Model file for the job. Use its own axes, mm. A direction names the side the tool comes from. Round coordinates to 2 decimals unless told otherwise and drop trailing zeros. Write each loop counter-clockwise with the first axis right and the second up, starting at its lowest first coordinate (ties: lowest second). Pieces come first, ordered by that corner, then holes. Notation, with made-up numbers: (30, 53.5) - (70, 53.5) arc R8 ccw to (70, 62.5) - close; hole circle Ø7 at (-24, 49). An arc over 180 degrees is marked (long way). One line per item, written item: value.
Autodesk Inventor part; units mm, degrees
ref_plane "作業平面1" through (2.15, -10, 1000) normal (0, 0, 1) x (1, 0, 0)
ref_plane "YZ Plane" through (0, 0, 0) normal (1, 0, 0) x (0, 1, 0)
ref_plane "XZ Plane" through (0, 0, 0) normal (0, 1, 0) x (-1, 0, 0)
ref_plane "作業平面1" through (2.15, -10, 1000) normal (0, 0, 1) x (1, 0, 0)
sketch "スケッチ1" plane through (2.15, -10, 1000) normal (0, 0, 1) x (1, 0, 0)
  line L0 (6.35, 12.15) -> (7.85, 12.15)
  line L1 (7.85, 12.15) -> (7.85, 19.4936)
  arc A0 (7.85, 19.4936) -> (7.3372, 19.9934) centre (7.35, 19.4936) ccw
  arc A1 (7.3372, 19.9934) -> (-12.1434, 0.5128) centre (7.85, 0) ccw
  arc A2 (-12.1434, 0.5128) -> (-11.6436, 0) centre (-11.6436, 0.5) ccw
  line L2 (-11.6436, 0) -> (-4.3, 0)
  line L3 (-4.3, 0) -> (-4.3, 1.5)
  line L4 (-4.3, 1.5) -> (-6.3, 1.5)
  line L5 (-6.3, 1.5) -> (-6.3, 5.2)
  line L6 (-6.3, 5.2) -> (-4.3, 5.2)
  line L7 (-4.3, 5.2) -> (-4.3, 7)
  line L8 (-4.3, 7) -> (0, 7)
  line L9 (0, 7) -> (0, 5.2)
  line L10 (0, 5.2) -> (2, 5.2)
  line L11 (2, 5.2) -> (2, 1.5)
  line L12 (2, 1.5) -> (0, 1.5)
  line L13 (0, 1.5) -> (0, 0)
  line L14 (0, 0) -> (7.35, 0)
  arc A3 (7.35, 0) -> (7.85, 0.5) centre (7.35, 0.5) ccw
  line L15 (7.85, 0.5) -> (7.85, 7.85)
  line L16 (7.85, 7.85) -> (6.35, 7.85)
  line L17 (6.35, 7.85) -> (6.35, 5.85)
  line L18 (6.35, 5.85) -> (2.65, 5.85)
  line L19 (2.65, 5.85) -> (2.65, 7.85)
  line L20 (2.65, 7.85) -> (0.85, 7.85)
  line L21 (0.85, 7.85) -> (0.85, 12.15)
  line L22 (0.85, 12.15) -> (2.65, 12.15)
  line L23 (2.65, 12.15) -> (2.65, 14.15)
  line L24 (2.65, 14.15) -> (6.35, 14.15)
  line L25 (6.35, 14.15) -> (6.35, 12.15)
  circle A4 centre (4.85, 3) radius 2
  circle A5 centre (-9.15, 3) radius 2
  circle A6 centre (4.85, 17) radius 2
  circle A7 centre (-2.15, 10) radius 1.65
extrude "押し出し1" add sketch "スケッチ1" along normal blind 40
properties part number "AFSR-2020-4-1000"
1. Tool access for faces 1 (the face through (4.8, 3, 1020)), 2 (the face through (2.15, -4, 1020)), 3 (the face through (4, -2.15, 1020)), 4 (the face through (2, 0, 1000)): list every direction of +Z, -Z, +X, -X, +Y, -Y with a clear straight run to the whole face (end or side of a thin tool).
Report:
face 1: +Z, -Z
face 2: +Z, -Z, -Y
face 3: +Z, -Z, +X
face 4: -Z, +X, -X, +Y, -Y
2. Band-saw the part on C-C on y = 0. Write the cut outline in (x, z), plus the area to 3 significant figures.
Report:
outline: (-7.32, 1000) - (-1.65, 1000) - (-1.65, 1040) - (-7.32, 1040) - close; (1.65, 1000) - (3, 1000) - (3, 1040) - (1.65, 1040) - close
area: 281 mm²
3. Band-saw the part on B-B on x = 7. Write the cut outline in (y, z).
Report:
outline: (-10, 1000) - (-9, 1000) - (-9, 1040) - (-10, 1040) - close; (-5, 1000) - (-4.15, 1000) - (-4.15, 1040) - (-5, 1040) - close; (4.15, 1000) - (5, 1000) - (5, 1040) - (4.15, 1040) - close; (9, 1000) - (9.77, 1000) - (9.77, 1040) - (9, 1040) - close
4. Band-saw the part on D-D on y = -7. Write the cut outline in (x, z).
Report:
outline: (-9.77, 1000) - (-9, 1000) - (-9, 1040) - (-9.77, 1040) - close; (-5, 1000) - (-4.15, 1000) - (-4.15, 1040) - (-5, 1040) - close; (4.15, 1000) - (5, 1000) - (5, 1040) - (4.15, 1040) - close; (9, 1000) - (10, 1000) - (10, 1040) - (9, 1040) - close
5. Band-saw the part on A-A on z = 1017.5. State how many separate pieces and enclosed holes the cut face has, plus the area to 3 significant figures.
Report:
separate pieces: 1
enclosed holes: 4
area: 178 mm²
6. Drop flat-ended pins along their axis: pin 1 (5 mm diameter, centred on y = -4, z = 1025.5, fed in from -X); pin 2 (1.4 mm diameter, centred on x = 4, z = 1030, fed in from +Y); pin 3 (1.6 mm diameter, centred on x = 2.5, z = 1027, fed in from +Y). Give the stop position or say it passes through.
Report:
pin 1: x = -9.69
pin 2: y = 9.28
pin 3: y = 8.84
7. Mould opens along X. For faces 5 (the face through (2.15, -9, 1020)), 6 (the face through (9, -2.15, 1020)), 7 (the face through (4.8, -3, 1020)), 8 (the face through (3, 0, 1020)) say: released by +X, released by -X, zero draft, split by the parting line, or undercut.
Report:
face 5: undercut
face 6: zero draft
face 7: undercut
face 8: released by +X
8. Wall check: probe 1 along Y at (x, z) = (7, 1009.5); probe 2 along Y at (x, z) = (7.5, 1036.5); probe 3 along X at (y, z) = (-7.75, 1020). Give the ranges that are in metal, low to high. Write a range as [from, to].
Report:
probe 1: [-10, -9], [-5, -4.15], [4.15, 5], [9, 9.77]
probe 2: [-10, -8.94], [-5.06, -4.15], [4.15, 5.06], [8.94, 9.84]
probe 3: [-9.87, -8.85], [-5.15, -4.15], [4.15, 5.15], [8.85, 10]
